Read the model definition and answer for the solid it produces. Units are mm, in the model's axes. Give positions to 0.01 mm unless a question says otherwise; leave off trailing zeros. Loops run counter-clockwise (first coordinate to the right, second up) from the corner with the lowest first, then second, coordinate; pieces in that order, holes last. Notation, with made-up numbers: (84, -0.75) -> (121, -0.75) arc R14 cw to (121, 5.25) -> close; hole circle Ø2 at (31, 65.5). An arc over 180 degrees is marked (long way). One line per item, written item: value. Start each with the question number.
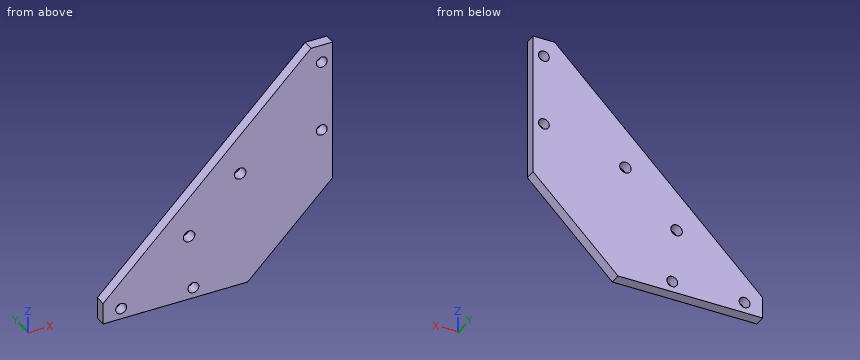
from build123d import *

# Parameters (mm, degrees)
SKETCH_1_R          = 1.5
EXTRUDE_1_DEPTH     = 3
SKETCH_2_R          = 1.6
CUT_EXTRUDE_1_DEPTH = 10


with BuildPart() as part:
    # 草图1 → 凸台-拉伸1 (new body)
    with BuildSketch(Plane(origin=(0, 0, 0), x_dir=(1, 0, 0), z_dir=(0, 1, 0))):
        Polygon((0, 0), (-40, 0), (-40, -6), (17.5, -63.5), (23.5, -63.5), (23.5, -23.5), align=None)
        with Locations(Location((-35, -3, 0), (0, 0, 270))):
            Circle(SKETCH_1_R, mode=Mode.SUBTRACT)
        with Locations(Location((-15, -3, 0), (0, 0, 270))):
            Circle(SKETCH_1_R, mode=Mode.SUBTRACT)
        with Locations(Location((20.5, -58.5, 0), (0, 0, 90))):
            Circle(SKETCH_1_R, mode=Mode.SUBTRACT)
        with Locations(Location((20.5, -38.5, 0), (0, 0, 90))):
            Circle(SKETCH_1_R, mode=Mode.SUBTRACT)
    extrude(amount=EXTRUDE_1_DEPTH)

    # 草图2 → 切除-拉伸1 (cut)
    with BuildSketch(Plane(origin=(0, 3, 0), x_dir=(1, 0, 0), z_dir=(0, 1, 0))):
        with Locations(Location((-16.199747468, -18.486544033, 0), (0, 0, 270))):
            Circle(SKETCH_2_R)
        with Locations(Location((-2.057611845, -32.628679656, 0), (0, 0, 270))):
            Circle(SKETCH_2_R)
    extrude(amount=-CUT_EXTRUDE_1_DEPTH, mode=Mode.SUBTRACT)


solid = part.part
Item 1: Section B-B, the plane x = -35 is taken. Determine the outline of the cut face in (y, z).
Item 2: Section C-C, the plane z = 38.5 is taken. Determine the outline of the cut face in (x, y), plus the area to 3 significant figures.
Item 3: Section A-A, the plane z = 3 is taken. Determine the outline of the cut face in (x, y).
Item 4: Consider L1, parallel to Z at x = 19.5, y = 1.5; L2, parallel to Z at x = 20.5, y = 1.8; L3, parallel to X at y = 1.8, z = 58.5. Determine where each line is inside the solid, lowest interval first. Write a range as [from, to].
Item 5: Section D-D, the plane x = 20.5 is taken. Determine the outline of the cut face in (y, z), plus the area to 3 significant figures.
Item 6: A flat-ended cylindrical pin translates along its axis: pin 1 (1.5 mm diameter, centred on y = 2, z = 46, fed in from -X). Find the tip coordinate at first contact, or state that the pin passes through.
Computed values:
1. outline: (0, 0) -> (3, 0) -> (3, 1.5) -> (0, 1.5) -> close; (0, 4.5) -> (3, 4.5) -> (3, 11) -> (0, 11) -> close
2. outline: (-7.5, 0) -> (19, 0) -> (19, 3) -> (-7.5, 3) -> close; (22, 0) -> (23.5, 0) -> (23.5, 3) -> (22, 3) -> close
2. area: 84.0 mm²
3. outline: (-40, 0) -> (-36.5, 0) -> (-36.5, 3) -> (-40, 3) -> close; (-33.5, 0) -> (-16.5, 0) -> (-16.5, 3) -> (-33.5, 3) -> close; (-13.5, 0) -> (3, 0) -> (3, 3) -> (-13.5, 3) -> close
4. L1: [19.5, 37.38], [39.62, 57.38], [59.62, 63.5]
4. L2: [20.5, 37], [40, 57], [60, 63.5]
4. L3: [12.5, 19], [22, 23.5]
5. outline: (0, 20.5) -> (3, 20.5) -> (3, 37) -> (0, 37) -> close; (0, 40) -> (3, 40) -> (3, 57) -> (0, 57) -> close; (0, 60) -> (3, 60) -> (3, 63.5) -> (0, 63.5) -> close
5. area: 111 mm²
6. pin 1: x = -0.75
